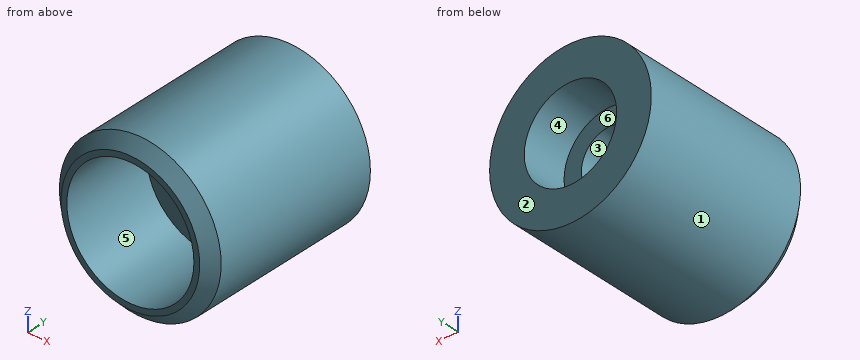
```python
from build123d import *

# Parameters (mm, degrees)
F0_R     = 7
F0_R_2   = 2.5
F1_DEPTH = 16
F2_R     = 4
F3_DEPTH = 4
F4_SIZE  = 1
F5_R     = 5.5
F6_DEPTH = 8


with BuildPart() as f1:
    # F0 (on Front) → F1 (new body)
    with BuildSketch(Plane.XZ):
        Circle(F0_R)
        Circle(F0_R_2, mode=Mode.SUBTRACT)
    extrude(amount=F1_DEPTH)

    # F2 (on Front) → F3 (cut)
    with BuildSketch(Plane.XZ):
        Circle(F2_R)
    extrude(amount=F3_DEPTH, mode=Mode.SUBTRACT)

    # F4
    f4_edges = [f1.edges().sort_by_distance(p)[0] for p in [
        (-7, -16, 0),
    ]]
    chamfer(f4_edges, length=F4_SIZE)

    # F2 (on Front) + F5 (on face) → F6 (cut)
    with BuildSketch(Plane.XZ):
        Circle(F2_R)
    with BuildSketch(Plane.XZ.offset(16)):
        Circle(F5_R)
    extrude(amount=-F6_DEPTH, mode=Mode.SUBTRACT)


solid = f1.part
```
Part model, mm, in its own coordinate system. Face numbers are marked on the shaded views. A direction names the side the tool comes from. Round coordinates to 2 decimals unless told otherwise and drop trailing zeros. Loops run counter-clockwise (first coordinate to the right, second up) from the corner with the lowest first, then second, coordinate; pieces in that order, holes last.
1. 3-axis set-ups, long thin cutter, end or side, ignore diameter. For the marked faces 5 and 6: which of +Z, -Z, +X, -X, +Y, -Y reach the whole face in a straight line?
Solutions:
face 5: -Y
face 6: +Y
2. Two-plate mould, pull along Z, no slides. Class the marked faces 1, 2, 3 and 4: pulls with the +Z half, pulls with the -Z half, needs draft (parallel to the pull), parting line crosses it, or undercut.
Solutions:
face 1: parting line crosses it
face 2: needs draft
face 3: undercut
face 4: undercut
3. Drill centre lines: line 1 along Z through (x, y) = (0, -11.5); line 2 along Z through (x, y) = (0, -5.5); line 3 along Y through (x, z) = (-2, -2.25). Where is each one in solid material? Low to high.
Solutions:
line 1: z = -7 to -5.5, 5.5 to 7
line 2: z = -7 to -2.5, 2.5 to 7
line 3: y = -8 to -4
4. Slice it at B-B (x = 0). Give the cut face in (y, z), and give its area (3 significant figures).
Solutions:
outline: (-16, -6) - (-15, -7) - (0, -7) - (0, -4) - (-4, -4) - (-4, -2.5) - (-8, -2.5) - (-8, -5.5) - (-16, -5.5) - close; (-16, 5.5) - (-8, 5.5) - (-8, 2.5) - (-4, 2.5) - (-4, 4) - (0, 4) - (0, 7) - (-15, 7) - (-16, 6) - close
area: 83.0 mm2
5. Flat gauge pins, fed straight in: pin 1 (5.5 mm diameter, centred on x = -1, z = 0, fed in from -Y); pin 2 (1 mm diameter, centred on y = -5, z = 5, fed in from +X); pin 3 (5 mm diameter, centred on y = -3, z = 4, fed in from +X). Where does each tip first touch, or does it go through?
Solutions:
pin 1: stops at y = -8
pin 2: stops at x = 5.36
pin 3: stops at x = 6.84
6. Slice it at C-C (y = -1.75). Give the cut face in (x, z).
Solutions:
outline: circle Ø14 at (0, 0); hole circle Ø8 at (0, 0)
7. Slice it at A-A (z = 0). Give the cut face in (x, y).
Solutions:
outline: (-7, -15) - (-6, -16) - (-5.5, -16) - (-5.5, -8) - (-2.5, -8) - (-2.5, -4) - (-4, -4) - (-4, 0) - (-7, 0) - close; (2.5, -8) - (5.5, -8) - (5.5, -16) - (6, -16) - (7, -15) - (7, 0) - (4, 0) - (4, -4) - (2.5, -4) - close
8. Slice it at D-D (y = -12). Give the cut face in (x, z).
Solutions:
outline: circle Ø14 at (0, 0); hole circle Ø11 at (0, 0)
